Check sheet for the modelled part. Datum: model origin and axes. Units: mm. Coordinates: 2 decimals unless noted, no trailing zeros. Loops run counter-clockwise (first coordinate to the right, second up) from the corner with the lowest first, then second, coordinate; pieces in that order, holes last. Notation, with made-up numbers: (51, 70.25) - (57, 70.25) arc R17 ccw to (57, 87.25) - close; hole circle Ø3 at (25, 60). An arc over 180 degrees is marked (long way). Use a Markdown table: item, result. Add a question column.
1) Sectioned sample at A-A, the plane x = 5. Enter the section's corners in (y, z).
2) Sectioned sample at C-C, the plane y = 2.35. State how many separate pieces and enclosed holes the cut face has, then the cut area to 3 significant figures.
3) Sectioned sample at D-D, the plane z = 20.5. Enter the section's corners in (x, y).
4) Go/stop test with a flat-tipped pin: P1, Ø1.2, axis at y = 2, z = -87.5, coming from the -X side. Record where the tip stops, or that it passes through.
5) Thickness scan on line 1 (X direction, y = 2.95, z = 30); line 2 (X direction, y = 0.35, z = -3.5); line 3 (Z direction, x = 97, y = 3.8). Record the ranges inside material, lowest first.
6) Sectioned sample at B-B, the plane z = 47. Enter the section's corners in (x, y).
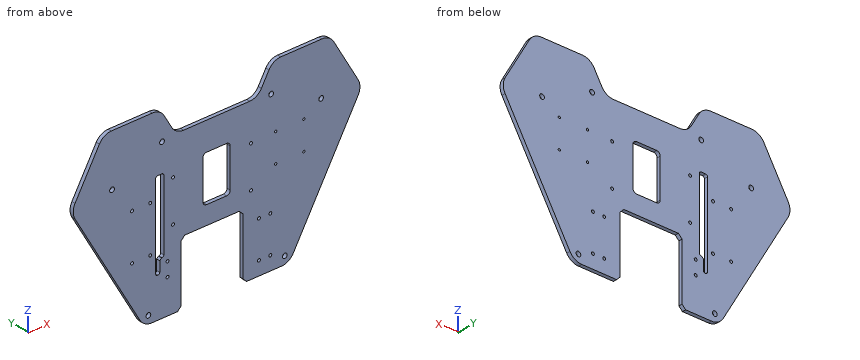
from build123d import *

# Parameters (mm, degrees)
EXTRUDE_1_DEPTH             = 4
SKETCH_34_R                 = 2.6
CUT_EXTRUDE_2_DEPTH         = 209.459490918
CUT_EXTRUDE_3_DEPTH         = 212.697897958
FILLET_2_R                  = 15
SKETCH_37_R                 = 1.6
CUT_EXTRUDE_5_DEPTH         = 210.949570549
PATTERN_LINEAR_1_COUNT      = 2
PATTERN_LINEAR_1_PITCH      = 85.74
PATTERN_LINEAR_1_COUNT_DIR2 = 2
PATTERN_LINEAR_1_PITCH_DIR2 = 45
SKETCH_38_R                 = 1.6
CUT_EXTRUDE_6_DEPTH         = 210.949570549
PATTERN_LINEAR_2_COUNT      = 2
PATTERN_LINEAR_2_PITCH      = 20
PATTERN_LINEAR_2_COUNT_DIR2 = 2
PATTERN_LINEAR_2_PITCH_DIR2 = 50
SKETCH_39_W                 = 68
SKETCH_39_H                 = 70
CUT_EXTRUDE_7_DEPTH         = 210.949570549
CHAMFER_1_SIZE              = 4
CUT_EXTRUDE_9_REACH         = 211.95
SKETCH_41_R                 = 1.6
SKETCH_42_R                 = 1.6
CUT_EXTRUDE_10_DEPTH        = 210.949570549
CUT_EXTRUDE_11_REACH        = 211.95
SKETCH_43_W                 = 30
SKETCH_43_H                 = 50
FILLET_3_R                  = 4
CUT_EXTRUDE_12_REACH        = 211.95
SKETCH_44_W                 = 9
SKETCH_44_H                 = 80
M3X0_5_1_D                  = 2.5
CUT_EXTRUDE_13_REACH        = 211.95
SKETCH_48_W                 = 4.5
SKETCH_48_H                 = 15
CHAMFER_2_SIZE              = 2
FILLET_8_R                  = 2


with BuildPart() as part:
    # 草圖1 → 填料-伸長1 (new body)
    with BuildSketch(Plane(origin=(0, 0, 0), x_dir=(1, 0, 0), z_dir=(0, 1, 0))):
        Polygon((124.529946162, -61.435935394), (-124.529946162, -61.435935394), (-160, 0), (-80, 138.564064606), (80, 138.564064606), (160, 0), align=None)
    extrude(amount=EXTRUDE_1_DEPTH)

    # 草圖34 → 除料-伸長2 (cut, through all)
    with BuildSketch(Plane(origin=(0, 4, -5), x_dir=(1, 0, 0), z_dir=(0, -1, 0))):
        with Locations(Location((-60, 35, 0), (0, 0, 270))):
            Circle(SKETCH_34_R)
        with Locations(Location((-115, 10, 0), (0, 0, 270))):
            Circle(SKETCH_34_R)
        with Locations(Location((-75, -125, 0), (0, 0, 270))):
            Circle(SKETCH_34_R)
    cut_extrude_2 = extrude(amount=CUT_EXTRUDE_2_DEPTH, mode=Mode.SUBTRACT)

    # 鏡射1: 除料-伸長2 across plane
    add(cut_extrude_2.mirror(Plane(origin=(0, 0, 0), x_dir=(0, 0, 1), z_dir=(1, 0, 0))), mode=Mode.SUBTRACT)

    # 草圖35 → 除料-伸長3 (cut, through all)
    with BuildSketch(Plane(origin=(0, 4, 0), x_dir=(1, 0, 0), z_dir=(0, 1, 0))):
        Polygon((45, -32.057713659), (-45, -32.057713659), (-90, -110), (-45, -187.942286341), (45, -187.942286341), (90, -110), align=None)
    extrude(amount=-CUT_EXTRUDE_3_DEPTH, mode=Mode.SUBTRACT)

    # 圓角2
    fillet_2_edges = [part.edges().sort_by_distance(p)[0] for p in [
        (160, 2, 0),
        (124.529946162, 2, 61.435935394),
        (-124.529946162, 2, 61.435935394),
        (-160, 2, 0),
        (-80, 2, -138.564064606),
        (80, 2, -138.564064606),
        (61.961524227, 2, 61.435935394),
        (45, 2, 32.057713659),
        (-61.961524227, 2, 61.435935394),
        (-45, 2, 32.057713659),
    ]]
    fillet(fillet_2_edges, radius=FILLET_2_R)

    # 草圖37 → 除料-伸長5 (cut, through all)
    with BuildSketch(Plane(origin=(0, 4, 0), x_dir=(1, 0, 0), z_dir=(0, 1, 0))):
        with Locations(Location((37.87, 8.564064606, 0), (0, 0, 270))):
            Circle(SKETCH_37_R)
    cut_extrude_5 = extrude(amount=-CUT_EXTRUDE_5_DEPTH, mode=Mode.SUBTRACT)

    # 直線複製排列1: Cut-Extrude 5 2 × 2
    with Locations(*[(-i * PATTERN_LINEAR_1_PITCH, 0, -j * PATTERN_LINEAR_1_PITCH_DIR2) for i in range(PATTERN_LINEAR_1_COUNT) for j in range(PATTERN_LINEAR_1_COUNT_DIR2) if (i, j) != (0, 0)]):
        add(cut_extrude_5, mode=Mode.SUBTRACT)

    # 草圖38 → 除料-伸長6 (cut, through all)
    with BuildSketch(Plane(origin=(0, 4, 0), x_dir=(1, 0, 0), z_dir=(0, 1, 0))):
        with Locations(Location((-73, 73.564064606, 0), (0, 0, 270))):
            Circle(SKETCH_38_R)
    cut_extrude_6 = extrude(amount=-CUT_EXTRUDE_6_DEPTH, mode=Mode.SUBTRACT)

    # 直線複製排列2: Cut-Extrude 6 2 × 2
    with Locations(*[(-i * PATTERN_LINEAR_2_PITCH, 0, j * PATTERN_LINEAR_2_PITCH_DIR2) for i in range(PATTERN_LINEAR_2_COUNT) for j in range(PATTERN_LINEAR_2_COUNT_DIR2) if (i, j) != (0, 0)]):
        add(cut_extrude_6, mode=Mode.SUBTRACT)

    # 草圖39 → 除料-伸長7 (cut, through all)
    with BuildSketch(Plane(origin=(0, 4, 0), x_dir=(1, 0, 0), z_dir=(0, 1, 0))):
        with Locations((-5, 103.564064606)):
            Rectangle(SKETCH_39_W, SKETCH_39_H)
    extrude(amount=-CUT_EXTRUDE_7_DEPTH, mode=Mode.SUBTRACT)

    # 導角1
    chamfer_1_edges = [part.edges().sort_by_distance(p)[0] for p in [
        (29, 2, -138.564064606),
        (29, 2, -68.564064606),
        (-39, 2, -68.564064606),
        (-39, 2, -138.564064606),
    ]]
    chamfer(chamfer_1_edges, length=CHAMFER_1_SIZE)

    # 草圖41 → 除料-伸長9 (cut, up to next)
    with BuildSketch(Plane(origin=(0, 4, 0), x_dir=(1, 0, 0), z_dir=(0, 1, 0)), mode=Mode.PRIVATE) as cut_extrude_9_sk1:
        with Locations(Location((59.1, 123.564064606, 0), (0, 0, 270))):
            Circle(SKETCH_41_R)
    cut_extrude_9_tool1 = extrude(cut_extrude_9_sk1.sketch, amount=-CUT_EXTRUDE_9_REACH, mode=Mode.PRIVATE) & part.part
    # 草圖41 → 除料-伸長9 (cut, up to next)
    with BuildSketch(Plane(origin=(0, 4, 0), x_dir=(1, 0, 0), z_dir=(0, 1, 0)), mode=Mode.PRIVATE) as cut_extrude_9_sk2:
        with Locations(Location((46.6, 123.564064606, 0), (0, 0, 270))):
            Circle(SKETCH_41_R)
    cut_extrude_9_tool2 = extrude(cut_extrude_9_sk2.sketch, amount=-CUT_EXTRUDE_9_REACH, mode=Mode.PRIVATE) & part.part
    # 草圖41 → 除料-伸長9 (cut, up to next)
    with BuildSketch(Plane(origin=(0, 4, 0), x_dir=(1, 0, 0), z_dir=(0, 1, 0)), mode=Mode.PRIVATE) as cut_extrude_9_sk3:
        with Locations(Location((46.6, 83.564064606, 0), (0, 0, 270))):
            Circle(SKETCH_41_R)
    cut_extrude_9_tool3 = extrude(cut_extrude_9_sk3.sketch, amount=-CUT_EXTRUDE_9_REACH, mode=Mode.PRIVATE) & part.part
    # 草圖41 → 除料-伸長9 (cut, up to next)
    with BuildSketch(Plane(origin=(0, 4, 0), x_dir=(1, 0, 0), z_dir=(0, 1, 0)), mode=Mode.PRIVATE) as cut_extrude_9_sk4:
        with Locations(Location((59.1, 83.564064606, 0), (0, 0, 270))):
            Circle(SKETCH_41_R)
    cut_extrude_9_tool4 = extrude(cut_extrude_9_sk4.sketch, amount=-CUT_EXTRUDE_9_REACH, mode=Mode.PRIVATE) & part.part
    add(cut_extrude_9_tool1.solids().sort_by_distance((59.1, 4, -123.564065))[0], mode=Mode.SUBTRACT)
    add(cut_extrude_9_tool2.solids().sort_by_distance((46.6, 4, -123.564065))[0], mode=Mode.SUBTRACT)
    add(cut_extrude_9_tool3.solids().sort_by_distance((46.6, 4, -83.564065))[0], mode=Mode.SUBTRACT)
    add(cut_extrude_9_tool4.solids().sort_by_distance((59.1, 4, -83.564065))[0], mode=Mode.SUBTRACT)

    # 草圖42 → 除料-伸長10 (cut, through all)
    with BuildSketch(Plane(origin=(0, 4, 0), x_dir=(1, 0, 0), z_dir=(0, 1, 0))):
        with Locations(Location((-54, 101.384064606, 0), (0, 0, 270))):
            Circle(SKETCH_42_R)
        with Locations(Location((-54, 86.384064606, 0), (0, 0, 270))):
            Circle(SKETCH_42_R)
    extrude(amount=-CUT_EXTRUDE_10_DEPTH, mode=Mode.SUBTRACT)

    # 草圖43 → 除料-伸長11 (cut, up to next)
    with BuildSketch(Plane(origin=(0, 4, 0), x_dir=(1, 0, 0), z_dir=(0, 1, 0)), mode=Mode.PRIVATE) as cut_extrude_11_sk1:
        with Locations((0, 23.564064606)):
            Rectangle(SKETCH_43_W, SKETCH_43_H)
    cut_extrude_11_tool1 = extrude(cut_extrude_11_sk1.sketch, amount=-CUT_EXTRUDE_11_REACH, mode=Mode.PRIVATE) & part.part
    add(cut_extrude_11_tool1.solids().sort_by_distance((0, 4, -23.564065))[0], mode=Mode.SUBTRACT)

    # 圓角3
    fillet_3_edges = [part.edges().sort_by_distance(p)[0] for p in [
        (15, 2, -48.564064606),
        (15, 2, 1.435935394),
        (-15, 2, 1.435935394),
        (-15, 2, -48.564064606),
    ]]
    fillet(fillet_3_edges, radius=FILLET_3_R)

    # 草圖44 → 除料-伸長12 (cut, up to next)
    with BuildSketch(Plane(origin=(0, 4, 0), x_dir=(1, 0, 0), z_dir=(0, 1, 0)), mode=Mode.PRIVATE) as cut_extrude_12_sk1:
        with Locations((-62.5, 40.564064606)):
            Rectangle(SKETCH_44_W, SKETCH_44_H)
    cut_extrude_12_tool1 = extrude(cut_extrude_12_sk1.sketch, amount=-CUT_EXTRUDE_12_REACH, mode=Mode.PRIVATE) & part.part
    add(cut_extrude_12_tool1.solids().sort_by_distance((-62.5, 4, -40.564065))[0], mode=Mode.SUBTRACT)

    # M3x0.5 螺紋孔1 (through all)
    with Locations(Plane(origin=(0, 4, 0), x_dir=(1, 0, 0), z_dir=(0, 1, 0))):
        with Locations((96, 7.564064606), (65, 7.564064606), (65, 38.564064606), (96, 38.564064606)):
            Hole(M3X0_5_1_D / 2)

    # 草圖48 → 除料-伸長13 (cut, up to next)
    with BuildSketch(Plane(origin=(0, 4, 0), x_dir=(1, 0, 0), z_dir=(0, 1, 0)), mode=Mode.PRIVATE) as cut_extrude_13_sk1:
        with Locations((-64.75, 88.064064606)):
            Rectangle(SKETCH_48_W, SKETCH_48_H)
    cut_extrude_13_tool1 = extrude(cut_extrude_13_sk1.sketch, amount=-CUT_EXTRUDE_13_REACH, mode=Mode.PRIVATE) & part.part
    add(cut_extrude_13_tool1.solids().sort_by_distance((-64.75, 4, -88.064065))[0], mode=Mode.SUBTRACT)

    # 導角2
    chamfer_2_edges = [part.edges().sort_by_distance(p)[0] for p in [
        (-62.5, 2, -80.564064606),
    ]]
    chamfer(chamfer_2_edges, length=CHAMFER_2_SIZE)

    # 圓角8
    fillet_8_edges = [part.edges().sort_by_distance(p)[0] for p in [
        (-58, 2, -80.564064606),
        (-58, 2, -0.564064606),
        (-67, 2, -0.564064606),
        (-62.5, 2, -95.564064606),
        (-67, 2, -95.564064606),
    ]]
    fillet(fillet_8_edges, radius=FILLET_8_R)


solid = part.part
Solved:
| question | item | result |
|---|---|---|
| 1 | outline | (0, -68.56) - (4, -68.56) - (4, -48.56) - (0, -48.56) - close; (0, 1.44) - (4, 1.44) - (4, 32.06) - (0, 32.06) - close |
| 2 | separate pieces | 1 |
| 2 | enclosed holes | 26 |
| 2 | area | 40,200 mm2 |
| 3 | outline | (-148.16, 0) - (148.16, 0) - (148.16, 4) - (-148.16, 4) - close |
| 4 | P1 | stops at x = -109.83 |
| 5 | line 1 | x = -142.68 to -62.6, -57.4 to 57.4, 62.6 to 142.68 |
| 5 | line 2 | x = -157.27 to -67, -58 to -15, 15 to 157.27 |
| 5 | line 3 | z = -109.12 to -39.31, -37.81 to -8.31, -6.81 to 61.44 |
| 6 | outline | (-132.86, 0) - (-53.63, 0) - (-53.63, 4) - (-132.86, 4) - close; (53.63, 0) - (132.86, 0) - (132.86, 4) - (53.63, 4) - close |
